Autodesk Inventor part; units mm, degrees
ref_plane "YZ Plane" through (0, 0, 0) normal (1, 0, 0) x (0, 1, 0)
ref_plane "XZ Plane" through (0, 0, 0) normal (0, 1, 0) x (-1, 0, 0)
ref_plane "XY Plane" through (0, 0, 0) normal (0, 0, 1) x (1, 0, 0)
sketch "スケッチ1" plane through (0, 0, 0) normal (0, 0, 1) x (1, 0, 0)
  line L0 (0, 0) -> (195, 0)
  line L1 (195, 0) -> (195, 170)
  line L2 (195, 170) -> (0, 170)
  line L3 (0, 170) -> (0, 0)
  line L4 (0, 0) -> (195, 170)
  dimension "d0" = 195
  dimension "d1" = 170
extrude "押し出し1" add sketch "スケッチ1" along normal blind 5 contours L3 L2 L4
sketch "スケッチ13" plane through (0, 0, 5) normal (0, 0, 1) x (1, 0, 0)
  line L0 (0, 0) -> (195, 170)
  line L1 (0, 0) -> (195, 170)
  line L2 (0, 0) -> (195, 170)
  line L3 (195, 170) -> (0, 170)
  line L4 (0, 170) -> (0, 0)
  line L5 (169.9396, 174.6857) -> (-13.756, 14.5408)
  line L6 (10, 160) -> (168.3118, 160)
  line L7 (168.3118, 160) -> (10, 21.9845)
  line L8 (10, 21.9845) -> (10, 160)
  point P0 (0, 26.5332)
  point P1 (164.5649, 170)
  point P2 (10, 35.2511)
  point P3 (153.0943, 160)
  dimension "d75" = 20
  dimension "d78" = 10
extrude "押し出し11" cut sketch "スケッチ13" against normal blind 10 contours L8 L6 L5
fillet "フィレット7" radius 5 3 edges at (10, 160, 2.5) (10, 35.2511, 2.5) (153.0943, 160, 2.5)
sketch "スケッチ14" plane through (0, 0, 5) normal (0, 0, 1) x (1, 0, 0)
  line L0 (15, 160) -> (139.7502, 160)
  arc A0 (143.0359, 151.2311) -> (139.7502, 160) centre (139.7502, 155) ccw
  line L1 (143.0359, 151.2311) -> (18.2857, 42.4746)
  arc A1 (10, 46.2434) -> (18.2857, 42.4746) centre (15, 46.2434) ccw
  line L2 (10, 46.2434) -> (10, 155)
  arc A2 (15, 160) -> (10, 155) centre (15, 155) ccw
  line L3 (0, 0) -> (195, 170)
  line L4 (195, 170) -> (0, 170)
  line L5 (0, 170) -> (0, 0)
  line L6 (164.5649, 170) -> (-7.7035, 19.8173)
  point P0 (143.0359, 151.2311)
  point P1 (0, 26.5332)
  point P2 (18.2857, 42.4746)
  dimension "d80" = 20
extrude "押し出し12" cut sketch "スケッチ14" against normal blind 10 contours A2 L2 A1 L6 L5 L4 A0 L0
properties part number "RP_Waist-Diagonal-material" material "A5052"
Input: part model. Units: mm. Frame: model coordinates. Round coordinates to 2 decimals unless told otherwise and drop trailing zeros. Loops run counter-clockwise (first coordinate to the right, second up) from the corner with the lowest first, then second, coordinate; pieces in that order, holes last.
1) Section query A-A on z = 1. Return the cut outline in (x, y).
Ans:
outline: (0, 0) - (195, 170) - (164.56, 170) - (18.29, 42.47) - (0, 26.53) - close
2) Material intervals for line 1 (X direction, y = 60, z = 1.1); line 2 (X direction, y = 104.5, z = 2.4); line 3 (Y direction, x = 159.5, z = 4.05), sorted ascending.
Ans:
line 1: x = 38.39 to 68.82
line 2: x = 89.43 to 119.87
line 3: y = 139.05 to 165.58
3) Pin query (flat end, axial travel): pin 1 (1.5 mm diameter, centred on y = 67.5, z = 3, fed in from +X); pin 2 (3 mm diameter, centred on y = 93, z = 1, fed in from +X); pin 3 (3 mm diameter, centred on x = 74, z = 4.5, fed in from -Y). Return the tip coordinate at first contact, or that it passes through.
Ans:
pin 1: stops at x = 78.29
pin 2: stops at x = 108.4
pin 3: stops at y = 63.21
4) Section query C-C on x = 14.5. Return the cut outline in (y, z), plus the area to 3 significant figures.
Ans:
outline: (12.64, 0) - (39.17, 0) - (39.17, 5) - (12.64, 5) - close
area: 133 mm2
5) Section query B-B on y = 20. Return the cut outline in (x, z), plus the area to 3 significant figures.
Ans:
outline: (0, 0) - (22.94, 0) - (22.94, 5) - (0, 5) - close
area: 115 mm2
